Design review of the part shown in the three views and the two pictorial views. Dimensions are in mm from the part's minimum x, y and z. A direction names the side the tool comes from. Round coordinates to 2 decimals unless told otherwise and drop trailing zeros. Loops run counter-clockwise (first coordinate to the right, second up) from the corner with the lowest first, then second, coordinate; pieces in that order, holes last. Notation, with made-up numbers: M 37.5,-9.75 L 75.5,-9.75 A14 ccw 75.5,15.25 Z; hole C 44.25,65.25 d3. An arc over 180 degrees is marked long. Return JSON: item names as keys, results as strings. Group by question number.
Q1. For the marked faces 1, 2, 3, 4 and 5, list the 3-axis set-ups (+Z, -Z, +X, -X, +Y, -Y) from which the entire face can be reached by the end or side of a thin tool; tool diameter is ignored.
Q2. Consider section C-C (x = 131). State the section outline as (y, z) points, and give its area (3 significant figures).
Q3. Draft analysis for pull direction X (two halves, no side actions). For the marked faces 6, 7 and 8, state which applies: pulls with the +X half, pulls with the -X half, needs draft (parallel to the pull), parting line crosses it, or undercut.
Q4. Clearance check with flat-ended pins moving along their axes: pin 1 Ø1 at (x, z) = (97, 24.5) entering from -Y; pin 2 Ø2 at (y, z) = (33, 52.5) entering from -X; pin 3 Ø6 at (x, z) = (23.5, 124.5) entering from +Y; pin 4 Ø1 at (y, z) = (37, 88) entering from +X. State where each tip first meets the part, or that it passes through.
Q5. Consider section D-D (y = 114). State the section outline as (x, z) points.
Q6. Consider section B-B (z = 120). State the section outline as (x, y) points (1 decimal), and give its area (3 significant figures).
Q7. To check wall thickness, follow line 1 along X through (y, z) = (116.5, 58.5); line 2 along Y through (x, z) = (29, 68.5); line 3 along Y through (x, z) = (82, 59.5). State the ranges of each line that lie inside material, in increasing order.
Q8. Consider section A-A (y = 64). State the section outline as (x, z) points.
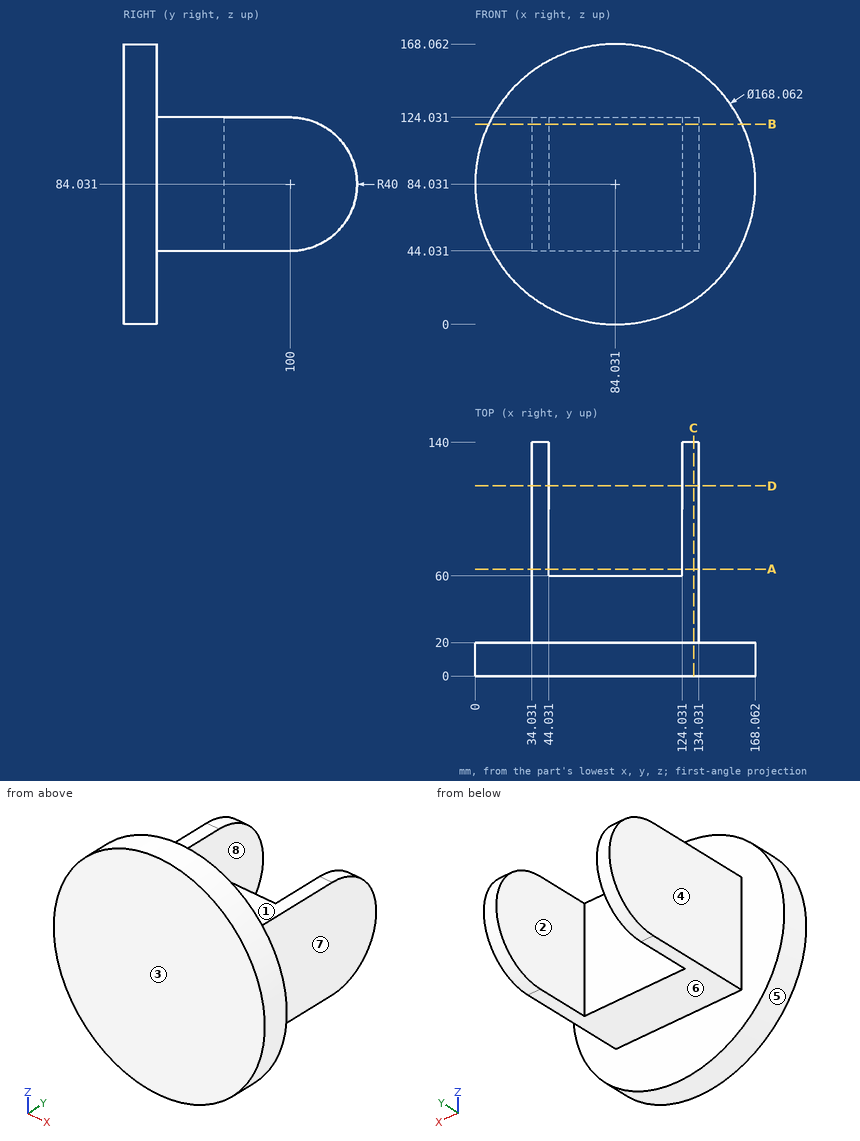
Values:
{
 "1": {"face 1": "+Z, +X, -X, +Y", "face 2": "+Z, -Z, +Y", "face 3": "+Z, -Z, +X, -X, -Y", "face 4": "+Z, -Z, -X, +Y", "face 5": "+Y, -Y"},
 "2": {"outline": "M 0,14.35 L 20,14.35 L 20,44.03 L 100,44.03 A40 ccw 100,124.03 L 20,124.03 L 20,153.71 L 0,153.71 Z", "area": "11,700 mm2"},
 "3": {"face 6": "needs draft", "face 7": "pulls with the +X half", "face 8": "undercut"},
 "4": {"pin 1": "stops at y = 0", "pin 2": "stops at x = 34.03", "pin 3": "stops at y = 20", "pin 4": "stops at x = 134.03"},
 "5": {"outline": "M 34.03,46.56 L 44.03,46.56 L 44.03,121.5 L 34.03,121.5 Z; M 124.03,46.56 L 134.03,46.56 L 134.03,121.5 L 124.03,121.5 Z"},
 "6": {"outline": "M 8.1,0 L 160,0 L 160,20 L 134,20 L 134,117.5 L 124,117.5 L 124,60 L 44,60 L 44,117.5 L 34,117.5 L 34,20 L 8.1,20 Z", "area": "8,190 mm2"},
 "7": {"line 1": "x = 34.03 to 44.03, 124.03 to 134.03", "line 2": "y = 0 to 20", "line 3": "y = 0 to 60"},
 "8": {"outline": "M 34.03,44.03 L 44.03,44.03 L 44.03,124.03 L 34.03,124.03 Z; M 124.03,44.03 L 134.03,44.03 L 134.03,124.03 L 124.03,124.03 Z"}
}
